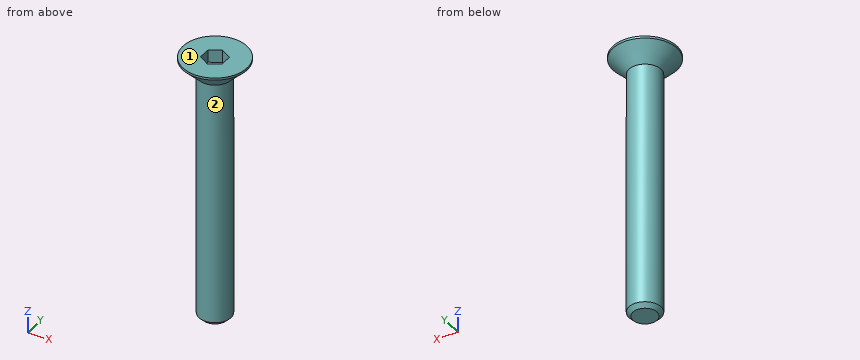
```python
from build123d import *

# Parameters (mm, degrees)
SKETCH1_W          = 25
SKETCH1_H          = 1.5
CHAMFER1_SIZE      = 0.375
CUT_EXTRUDE2_DEPTH = 1.19


with BuildPart() as part:
    # Sketch1 → Revolve1 (revolve)
    with BuildSketch(Plane(origin=(0, 0, 0), x_dir=(0, 0, -1), z_dir=(1, 0, 0))):
        with Locations((12.5, 0.75)):
            Rectangle(SKETCH1_W, SKETCH1_H)
    revolve(axis=Axis((0, 0, -25), (0, 0, 1)))

    # Chamfer1
    chamfer1_edges = [part.edges().sort_by_distance(p)[0] for p in [
        (0, -1.5, -25),
    ]]
    chamfer(chamfer1_edges, length=CHAMFER1_SIZE)

    # Sketch7 → Revolve2 (revolve)
    with BuildSketch(Plane(origin=(0, 0, 0), x_dir=(0, 0, -1), z_dir=(1, 0, 0)), mode=Mode.PRIVATE) as revolve2_sk:
        Polygon((0, 3), (0.2, 3), (1.7, 1.5), (1.7, 0), (0, 0), align=None)
    revolve(revolve2_sk.sketch.rotate(Axis((0, 0, 0), (0, 0, -1)), 180), axis=Axis((0, 0, 0), (0, 0, -1)))

    # Boss-Extrude1 cone 1 section (through the dimple's axis) → Boss-Extrude1 (revolve)
    with BuildSketch(Plane(origin=(0, 0, -1.7), x_dir=(0, -1, 0), z_dir=(1, 0, 0))):
        Polygon((0, 0), (1.5, 0), (0, 1.5), align=None)
    revolve(axis=Axis((0, 0, -1.7), (0, 0, -1)))

    # Sketch5 → Cut-Extrude2 (cut)
    with BuildSketch(Plane.XY):
        Polygon((1, -0.577350269), (1, 0.577350269), (0, 1.154700538), (-1, 0.577350269), (-1, -0.577350269), (0, -1.154700538), align=None)
    extrude(amount=-CUT_EXTRUDE2_DEPTH, mode=Mode.SUBTRACT)


solid = part.part
```
Work out the finished part from the listing and answer in its coordinate system (mm). Face numbers are marked on the shaded views. A direction names the side the tool comes from. Give positions to 0.01 mm unless a question says otherwise; leave off trailing zeros. Loops run counter-clockwise (first coordinate to the right, second up) from the corner with the lowest first, then second, coordinate; pieces in that order, holes last. Notation, with made-up numbers: (-18, 13.5) -> (40, 13.5) arc R27 ccw to (40, 51.5) -> close; hole circle Ø8 at (-38, -16). An arc over 180 degrees is marked (long way). One line per question, with ' | ' between items. Start each with the question number.
1) For the marked faces 1 and 2, determine the directions among +Z, -Z, +X, -X, +Y, -Y from which every point of the face is accessible in a straight line to the end or side of a thin tool.
2) Section A-A, the plane y = 0 is taken. Determine the outline of the cut face in (x, z) (3 decimals), then the cut area to 3 significant figures.
3) Section B-B, the plane z = -21.75 is taken. Determine the outline of the cut face in (x, y), then the cut area to 3 significant figures.
4) Each of these flat-tipped pins is pushed along its axis until it touches: pin 1 (1 mm diameter, centred on x = -1, y = -2, fed in from -Z); pin 2 (1.3 mm diameter, centred on y = 0, z = -0.5, fed in from -X); pin 3 (1 mm diameter, centred on x = 1, z = -12, fed in from +Y). Where does it stop, or does it pass through?
5) Straight lines are drawn through the part: L1, parallel to Z at x = -1.55, y = 0.7; L2, parallel to Z at x = 0.6, y = -0.45; L3, parallel to X at y = 0.95, z = -2.25. For each, find the intervals that lie inside material, in ascending order.
Resolved:
1) face 1: +Z, +X, -X, +Y, -Y | face 2: -Z
2) outline: (-3, -0.2) -> (-1.5, -1.7) -> (-1.5, -24.625) -> (-1.125, -25) -> (1.125, -25) -> (1.5, -24.625) -> (1.5, -1.7) -> (3, -0.2) -> (3, 0) -> (1, 0) -> (1, -1.19) -> (-1, -1.19) -> (-1, 0) -> (-3, 0) -> close | area: 75.3 mm2
3) outline: circle Ø3 at (0, 0) | area: 7.07 mm2
4) pin 1: z = -1.46 | pin 2: x = -3 | pin 3: y = 1.41
5) L1: -1.5 to 0 | L2: -25 to -1.19 | L3: -1.16 to 1.16
